The listing builds one solid part. Answer for the finished solid, in the listing's coordinates (mm). Face numbers are marked on the shaded views. A direction names the side the tool comes from. Give positions to 0.01 mm unless a question says otherwise; leave off trailing zeros. Loops run counter-clockwise (first coordinate to the right, second up) from the corner with the lowest first, then second, coordinate; pieces in that order, holes last.
Item 1: Section B-B, the plane z = 4.5 is taken. Give the vertices of the cut face in (x, y).
Item 2: Section A-A, the plane y = 0 is taken. Give the vertices of the cut face in (x, z).
Item 3: Section D-D, the plane z = 15 is taken. Give the vertices of the cut face in (x, y), and give its area (3 significant figures).
Item 4: Consider line 1 along X through (y, z) = (5.85, 2.5); line 2 along Y through (x, z) = (0, 15.25); line 3 along Z through (x, y) = (0, 4.95). Determine where each line is inside the solid, lowest interval first.
Item 5: Each of these flat-tipped pins is pushed along its axis until it touches: pin 1 Ø4 at (y, z) = (4.5, 7) entering from +X; pin 2 Ø6 at (x, z) = (4, 11.5) entering from -Y; pin 3 Ø5.5 at (x, y) = (-3, 0.5) entering from -Z. Where does it stop, or does it pass through?
Item 6: The mould has two halves that part along Z. Classify the marked faces 1, 2 and 3: pulls with the +Z half, pulls with the -Z half, needs draft (parallel to the pull), parting line crosses it, or undercut.
Item 7: Section C-C, the plane x = -3 is taken. Give the vertices of the cut face in (y, z).
Item 8: A tool of negligible diameter and unlimited length cuts with its end or side. For the marked faces 4 and 5, from which of +Z, -Z, +X, -X, +Y, -Y can it reach the whole face along a straight path? Write none if from no direction.
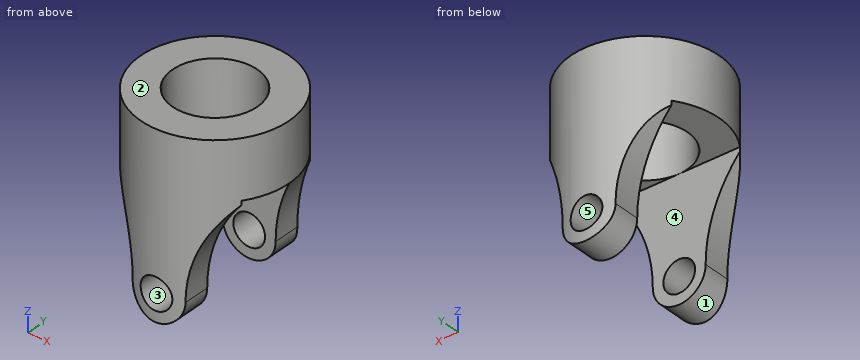
from build123d import *

# Parameters (mm, degrees)
SKETCH1_R               = 7
SKETCH1_R_2             = 4
BOSS_EXTRUDE1_DEPTH     = 17
SKETCH2_R               = 1.5
CUT_EXTRUDE1_DEPTH      = 8
CUT_EXTRUDE1_DEPTH_BACK = 8
SKETCH3_W               = 11.5
SKETCH3_H               = 8
CUT_EXTRUDE2_DEPTH      = 8.0000001
CUT_EXTRUDE2_DEPTH_BACK = 8.0000001


with BuildPart() as part:
    # Sketch1 → Boss-Extrude1 (new body)
    with BuildSketch(Plane.XY):
        Circle(SKETCH1_R)
        Circle(SKETCH1_R_2, mode=Mode.SUBTRACT)
    extrude(amount=BOSS_EXTRUDE1_DEPTH)

    # Sketch2 → Cut-Extrude1 (cut, two sides)
    with BuildSketch(Plane(origin=(0, 0, 0), x_dir=(1, 0, 0), z_dir=(0, 1, 0))) as cut_extrude1_sk:
        with Locations((0, -2.5)):
            Circle(SKETCH2_R)
        with BuildLine():
            Line((-7, -11.5), (-7, 0))
            Line((-7, 0), (0, 1))
            Line((0, 1), (7, 0))
            Line((7, 0), (7, -11.5))
            Line((7, -11.5), (6.109441797, -11.5))
            ThreePointArc((6.109441797, -11.5), (3.435990323, -7.348403606), (2.5, -2.5))
            ThreePointArc((2.5, -2.5), (0, 0), (-2.5, -2.5))
            ThreePointArc((-2.5, -2.5), (-3.435990323, -7.348403606), (-6.109441797, -11.5))
            Line((-6.109441797, -11.5), (-7, -11.5))
        make_face()
    extrude(amount=CUT_EXTRUDE1_DEPTH, mode=Mode.SUBTRACT)
    extrude(cut_extrude1_sk.sketch, amount=-CUT_EXTRUDE1_DEPTH_BACK, mode=Mode.SUBTRACT)

    # Sketch3 → Cut-Extrude2 (cut, two sides)
    with BuildSketch(Plane(origin=(0, 0, 0), x_dir=(0, 0, -1), z_dir=(1, 0, 0))) as cut_extrude2_sk:
        with Locations((-5.75, 0)):
            Rectangle(SKETCH3_W, SKETCH3_H)
    extrude(amount=CUT_EXTRUDE2_DEPTH, mode=Mode.SUBTRACT)
    extrude(cut_extrude2_sk.sketch, amount=-CUT_EXTRUDE2_DEPTH_BACK, mode=Mode.SUBTRACT)


solid = part.part
Worked answers:
1. outline: (-2.65, -6.48) arc R7 ccw to (2.65, -6.48) - (2.65, -4) - (-2.65, -4) - close; (-2.65, 4) - (2.65, 4) - (2.65, 6.48) arc R7 ccw to (-2.65, 6.48) - close
2. outline: (-7, 11.5) - (-4, 11.5) - (-4, 17) - (-7, 17) - close; (4, 11.5) - (7, 11.5) - (7, 17) - (4, 17) - close
3. outline: circle Ø14 at (0, 0); hole circle Ø8 at (0, 0)
3. area: 104 mm2
4. line 1: x = -2.5 to -1.5, 1.5 to 2.5
4. line 2: y = -7 to -4, 4 to 7
4. line 3: z = 0 to 1, 4 to 17
5. pin 1: stops at x = 4.24
5. pin 2: stops at y = -6.93
5. pin 3: stops at z = 11.5
6. face 1: pulls with the -Z half
6. face 2: pulls with the +Z half
6. face 3: undercut
7. outline: (-6.32, 6.07) - (-4, 6.07) - (-4, 11.5) - (-2.65, 11.5) - (-2.65, 17) - (-6.32, 17) - close; (2.65, 11.5) - (4, 11.5) - (4, 6.07) - (6.32, 6.07) - (6.32, 17) - (2.65, 17) - close
8. face 4: -Z, +X, -X
8. face 5: +Y, -Y
